The figure shows three views and two pictorial views of one solid part (mm, origin at its lowest corner). Answer the questions. A direction names the side the tool comes from. Round coordinates to 2 decimals unless told otherwise and drop trailing zeros. Write each loop counter-clockwise with the first axis right and the second up, starting at its lowest first coordinate (ties: lowest second). Pieces come first, ordered by that corner, then holes. Notation, with made-up numbers: (-5.75, 62.5) - (12.25, 62.5) arc R21 ccw to (12.25, 83.5) - close; hole circle Ø11 at (69, 43.25). An arc over 180 degrees is marked (long way). Answer as CSV lines item,"result". Start each with the question number.
Item 1: A cutting plane is placed at C-C on y = 7. Determine the outline of the cut face in (x, z), and give its area (3 significant figures).
Item 2: A cutting plane is placed at D-D on x = 70. Determine the outline of the cut face in (y, z).
Item 3: Flat-ended cylindrical pins translate along their axes: pin 1 (11.5 mm diameter, centred on y = 58.5, z = 28, fed in from +X); pin 2 (16 mm diameter, centred on x = 18.5, y = 41.5, fed in from -Z); pin 3 (12 mm diameter, centred on x = 61.5, y = 7, fed in from +Z). Find the tip coordinate at first contact, or state that the pin passes through.
Item 4: A cutting plane is placed at B-B on x = 55. Determine the outline of the cut face in (y, z).
Item 5: Which of the six approach directions +Z, -Z, +X, -X, +Y, -Y give full straight-line access (tool end or side, diameter ignored) to the marked faces 1, 2 and 3?
Item 6: Straight lines are drawn through the part: line 1 along Z through (x, y) = (35.5, 17); line 2 along Z through (x, y) = (51, 38); line 3 along X through (y, z) = (30, 34.5) (1 decimal). For each, find the intervals that lie inside material, in ascending order. Write a range as [from, to].
Item 7: A cutting plane is placed at A-A on y = 57. Determine the outline of the cut face in (x, z), and give its area (3 significant figures).
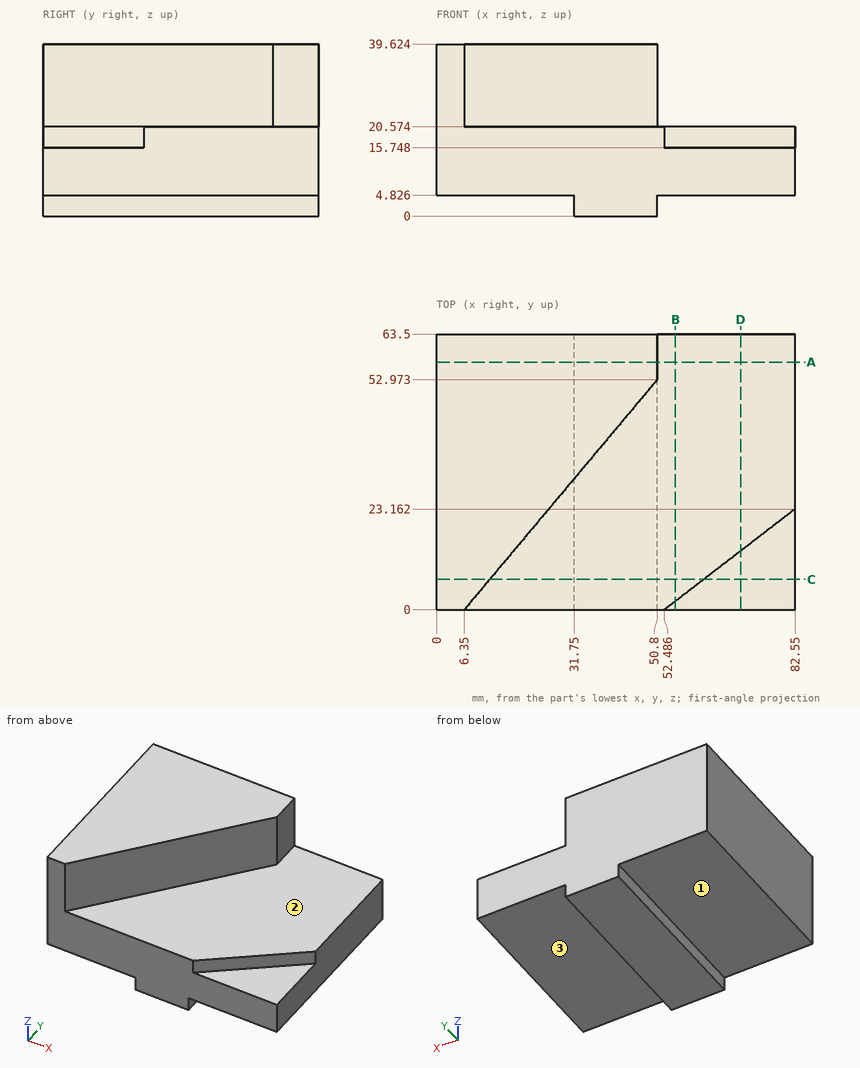
Geometry says:
1,outline,"(0, 4.83) - (31.75, 4.83) - (31.75, 0) - (50.8, 0) - (50.8, 4.83) - (82.55, 4.83) - (82.55, 15.75) - (61.57, 15.75) - (61.57, 20.57) - (12.22, 20.57) - (12.22, 39.62) - (0, 39.62) - close"
1,area,"1,520 mm^2"
2,outline,"(0, 4.83) - (63.5, 4.83) - (63.5, 20.57) - (13.49, 20.57) - (13.49, 15.75) - (0, 15.75) - close"
3,pin 1,"stops at x = 50.8"
3,pin 2,"stops at z = 4.83"
3,pin 3,"stops at z = 20.57"
4,outline,"(0, 4.83) - (63.5, 4.83) - (63.5, 20.57) - (1.94, 20.57) - (1.94, 15.75) - (0, 15.75) - close"
5,face 1,"-Z, -X, +Y, -Y"
5,face 2,"+Z, +X, -Y"
5,face 3,"-Z, +X, +Y, -Y"
6,line 1,"z = [0, 20.57]"
6,line 2,"z = [4.83, 20.57]"
6,line 3,"x = [0, 31.5]"
7,outline,"(0, 4.83) - (31.75, 4.83) - (31.75, 0) - (50.8, 0) - (50.8, 4.83) - (82.55, 4.83) - (82.55, 20.57) - (50.8, 20.57) - (50.8, 39.62) - (0, 39.62) - close"
7,area,"2,360 mm^2"
